Autodesk Inventor part; units mm, degrees
ref_plane "p1_XY" through (0, 0, 4.7816) normal (1, 0, 0) x (0, 0, -1)
ref_plane "p1_YZ" through (0, 0, 4.7816) normal (0, 0, -1) x (0, 1, 0)
ref_plane "p1_ZX" through (0, 0, 4.7816) normal (0, 1, 0) x (1, 0, 0)
sketch "Sketch_1" plane through (0, 0, 0) normal (0, 0, 1) x (1, 0, 0)
  line L0 (13.0937, 0) -> (-13.0937, 0)
  line L1 (-13.0937, 0) -> (-13.0937, 4.4005)
  line L2 (-13.0937, 4.4005) -> (-12.7127, 4.7816)
  line L3 (-12.7127, 4.7816) -> (-10.6172, 4.7816)
  line L4 (-10.6172, 4.7816) -> (-10.6172, 3.8672)
  line L5 (-10.6172, 3.8672) -> (-9.5885, 3.8672)
  line L6 (-9.5885, 3.8672) -> (-9.5885, 4.7816)
  line L7 (-9.5885, 4.7816) -> (9.5885, 4.7816)
  line L8 (9.5885, 4.7816) -> (9.5885, 3.8672)
  line L9 (9.5885, 3.8672) -> (10.6172, 3.8672)
  line L10 (10.6172, 3.8672) -> (10.6172, 4.7816)
  line L11 (10.6172, 4.7816) -> (12.7127, 4.7816)
  line L12 (12.7127, 4.7816) -> (13.0937, 4.4005)
  line L13 (13.0937, 4.4005) -> (13.0937, 0)
  line L14 (13.0937, 0) -> (-13.0937, 0)
revolve "Revolution1" add sketch "Sketch_1" angle 360 about axis through (13.0937, 0, 0) along (1, 0, 0)
ref_plane "p1_XY" through (0, 0, 4.7816) normal (1, 0, 0) x (0, 0, -1)
ref_plane "p1_YZ" through (0, 0, 4.7816) normal (0, 0, -1) x (0, 1, 0)
ref_plane "p1_ZX" through (0, 0, 4.7816) normal (0, 1, 0) x (1, 0, 0)
ref_plane "p2_XY" through (0, 0, -4.7816) normal (1, 0, 0) x (0, 0, -1)
ref_plane "p2_YZ" through (0, 0, -4.7816) normal (0, 0, -1) x (0, 1, 0)
ref_plane "p2_ZX" through (0, 0, -4.7816) normal (0, 1, 0) x (1, 0, 0)
ref_plane "pin_XY" through (0, 0, 0) normal (1, 0, 0) x (0, 0, -1)
ref_plane "pin_YZ" through (0, 0, 0) normal (0, 0, -1) x (0, 1, 0)
ref_plane "pin_ZX" through (0, 0, 0) normal (0, 1, 0) x (1, 0, 0)
ref_plane "rr1_XY" through (10.1029, 0, 0) normal (1, 0, 0) x (0, 0, -1)
ref_plane "rr1_YZ" through (10.1029, 0, 0) normal (0, 0, -1) x (0, 1, 0)
ref_plane "rr1_ZX" through (10.1029, 0, 0) normal (0, 1, 0) x (1, 0, 0)
ref_plane "rr2_XY" through (-10.1029, 0, 0) normal (1, 0, 0) x (0, 0, -1)
ref_plane "rr2_YZ" through (-10.1029, 0, 0) normal (0, 0, -1) x (0, 1, 0)
ref_plane "rr2_ZX" through (-10.1029, 0, 0) normal (0, 1, 0) x (1, 0, 0)
ref_plane "w21_XY" through (13.0937, 0, 0) normal (0, 1, 0) x (1, 0, 0)
ref_plane "w21_YZ" through (13.0937, 0, 0) normal (1, 0, 0) x (0, 0, -1)
ref_plane "w21_ZX" through (13.0937, 0, 0) normal (0, 0, -1) x (0, 1, 0)
ref_plane "w22_XY" through (-13.0937, 0, 0) normal (0, 1, 0) x (1, 0, 0)
ref_plane "w22_YZ" through (-13.0937, 0, 0) normal (1, 0, 0) x (0, 0, -1)
ref_plane "w22_ZX" through (-13.0937, 0, 0) normal (0, 0, -1) x (0, 1, 0)
equation "\"BendRadius\" = Thickness"
equation "\"BendReliefWidth\" = Thickness"
equation "\"BendReliefDepth\" = 0.5 * Thickness"
equation "\"CornerReliefSize\" = 4 * Thickness"
equation "\"MinimumRemnant\" = 2 * Thickness"
equation "\"TransitionRadius\" = BendRadius"
equation "\"JacobiRadiusSize\" = Thickness"
equation "\"GapSize\" = Thickness"
properties part number "D-8383"
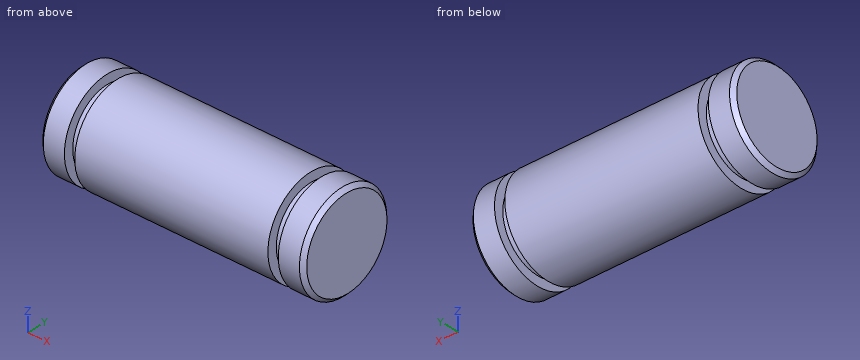
Part model, mm, in its own coordinate system. Round coordinates to 2 decimals unless told otherwise and drop trailing zeros. Loops run counter-clockwise (first coordinate to the right, second up) from the corner with the lowest first, then second, coordinate; pieces in that order, holes last.
Item 1: Drop a flat-ended pin along its axis: P1, Ø3, axis at y = -3.5, z = 3.5, coming from the +X side. Give the stop position or say it passes through.
Item 2: Cut at A-A, the plane z = 0. Give the cut face in (x, y).
Item 3: Drill centre lines: line 1 (X direction, y = 2, z = 3.5); line 2 (Y direction, x = 6.25, z = 4.25); line 3 (Z direction, x = -0.75, y = 3.75). Where is each one in solid material? Low to high.
Item 4: Cut at C-C, the plane x = 6.5. Give the cut face in (y, z).
A:
1. P1: stops at x = 13.09
2. outline: (-13.09, -4.4) - (-12.71, -4.78) - (-10.62, -4.78) - (-10.62, -3.87) - (-9.59, -3.87) - (-9.59, -4.78) - (9.59, -4.78) - (9.59, -3.87) - (10.62, -3.87) - (10.62, -4.78) - (12.71, -4.78) - (13.09, -4.4) - (13.09, 4.4) - (12.71, 4.78) - (10.62, 4.78) - (10.62, 3.87) - (9.59, 3.87) - (9.59, 4.78) - (-9.59, 4.78) - (-9.59, 3.87) - (-10.62, 3.87) - (-10.62, 4.78) - (-12.71, 4.78) - (-13.09, 4.4) - close
3. line 1: x = -13.09 to -10.62, -9.59 to 9.59, 10.62 to 13.09
3. line 2: y = -2.19 to 2.19
3. line 3: z = -2.97 to 2.97
4. outline: circle Ø9.56 at (0, 0)
